```python
from build123d import *

# Parameters (mm, degrees)
BASE_PLATE_R        = 1.6
EXTRUDE_1_DEPTH     = 6
CUT_EXTRUDE_START   = -6
SKETCH_1_R          = 3.25
SKETCH_1_R_2        = 3.5
CUT_EXTRUDE_1_DEPTH = 4.5
SKETCH_1_6_R        = 2.4
CUT_EXTRUDE_2_DEPTH = 2
SKETCH_1_7_R        = 2.5
CUT_EXTRUDE_3_DEPTH = 1.4
FILLET_2_R          = 0.5


with BuildPart() as part:
    # Base plate → 凸台-拉伸1 (new body)
    with BuildSketch(Plane(origin=(0, 0, 0), x_dir=(1, 0, 0), z_dir=(0, 1, 0))):
        with BuildLine():
            Line((-38.1, -38.1), (38.1, -38.1))
            Line((38.1, -38.1), (38.1, 38.1))
            Line((38.1, 38.1), (-0.9, 38.1))
            Line((-0.9, 38.1), (-0.9, 27.4))
            ThreePointArc((-0.9, 27.4), (-2.9, 25.4), (-4.9, 27.4))
            Line((-4.9, 27.4), (-4.9, 38.1))
            Line((-4.9, 38.1), (-38.1, 38.1))
            Line((-38.1, 38.1), (-38.1, -38.1))
        make_face()
        with Locations(Location((-33.9, -33.9, 0), (0, 0, 270))):
            Circle(BASE_PLATE_R, mode=Mode.SUBTRACT)
        with Locations(Location((33.9, -33.9, 0), (0, 0, 270))):
            Circle(BASE_PLATE_R, mode=Mode.SUBTRACT)
        with Locations(Location((-33.9, 33.9, 0), (0, 0, 270))):
            Circle(BASE_PLATE_R, mode=Mode.SUBTRACT)
        with Locations(Location((33.9, 33.9, 0), (0, 0, 270))):
            Circle(BASE_PLATE_R, mode=Mode.SUBTRACT)
    extrude(amount=EXTRUDE_1_DEPTH)

    # 草图1 → 切除-拉伸1 (cut)
    with BuildSketch(Plane.XZ.offset(CUT_EXTRUDE_START)):
        with Locations(Location((-0.35, 10.415, 0), (0, 0, 90))):
            Circle(SKETCH_1_R)
        with Locations(Location((-22.7, 23.9, 0), (0, 0, 90))):
            Circle(SKETCH_1_R)
        with Locations(Location((-22.7, -3.07, 0), (0, 0, 90))):
            Circle(SKETCH_1_R)
        with Locations(Location((-17.96, -15.36, 0), (0, 0, 90))):
            Circle(SKETCH_1_R_2)
        with Locations(Location((-5.01, -15.36, 0), (0, 0, 90))):
            Circle(SKETCH_1_R_2)
    extrude(amount=CUT_EXTRUDE_1_DEPTH, mode=Mode.SUBTRACT)

    # 草图1<6> → 切除-拉伸2 (cut)
    with BuildSketch(Plane.XZ.offset(CUT_EXTRUDE_START)):
        with BuildLine():
            Line((8.9, 2), (8.9, -7.4))
            ThreePointArc((8.9, -7.4), (11.4, -9.9), (13.9, -7.4))
            Line((13.9, -7.4), (13.9, 2))
            ThreePointArc((13.9, 2), (11.4, 4.5), (8.9, 2))
        make_face()
        with BuildLine():
            Line((21.6, -0.16), (21.6, -5.24))
            ThreePointArc((21.6, -5.24), (24.1, -7.74), (26.6, -5.24))
            Line((26.6, -5.24), (26.6, -0.16))
            ThreePointArc((26.6, -0.16), (24.1, 2.34), (21.6, -0.16))
        make_face()
        with Locations(Location((31.9, -15.1, 0), (0, 0, 90))):
            Circle(SKETCH_1_6_R)
        with Locations(Location((16.7, -15.1, 0), (0, 0, 90))):
            Circle(SKETCH_1_6_R)
    extrude(amount=CUT_EXTRUDE_2_DEPTH, mode=Mode.SUBTRACT)

    # 草图1<7> → 切除-拉伸3 (cut)
    with BuildSketch(Plane.XZ.offset(CUT_EXTRUDE_START)):
        with BuildLine():
            Line((17.15, -38.1), (21.65, -38.1))
            Line((21.65, -38.1), (21.65, -37.1))
            Line((21.65, -37.1), (21.65, -36.1))
            ThreePointArc((21.65, -36.1), (20.560909108, -34.172620939), (18.347964405, -34.111100529))
            ThreePointArc((18.347964405, -34.111100529), (17.472620939, -34.939090892), (17.15, -36.1))
            Line((17.15, -36.1), (17.15, -38.1))
        make_face()
        with BuildLine():
            Line((21.65, -36.1), (21.65, -37.1))
            Line((21.65, -37.1), (25.452035595, -35.088899471))
            ThreePointArc((25.452035595, -35.088899471), (23.239090892, -35.027379061), (22.15, -33.1))
            Line((22.15, -33.1), (22.15, -32.1))
            Line((22.15, -32.1), (18.347964405, -34.111100529))
            ThreePointArc((18.347964405, -34.111100529), (20.560909108, -34.172620939), (21.65, -36.1))
        make_face()
        with BuildLine():
            ThreePointArc((22.15, -33.1), (24.4, -35.35), (26.65, -33.1))
            Line((26.65, -33.1), (26.65, -28.1))
            ThreePointArc((26.65, -28.1), (24.4, -25.85), (22.15, -28.1))
            Line((22.15, -28.1), (22.15, -33.1))
        make_face()
        with BuildLine():
            Line((18.347964405, -27.088899471), (22.15, -29.1))
            Line((22.15, -29.1), (22.15, -28.1))
            ThreePointArc((22.15, -28.1), (23.239090892, -26.172620939), (25.452035595, -26.111100529))
            Line((25.452035595, -26.111100529), (22.211102988, -24.396797462))
            Line((22.211102988, -24.396797462), (21.438912065, -26.051492297))
            ThreePointArc((21.438912065, -26.051492297), (20.115915291, -27.233064766), (18.347964405, -27.088899471))
        make_face()
        with BuildLine():
            Line((18.761087935, -21.148507703), (17.361087935, -24.148507703))
            ThreePointArc((17.361087935, -24.148507703), (18.448507703, -27.138912065), (21.438912065, -26.051492297))
            Line((21.438912065, -26.051492297), (22.838912065, -23.051492297))
            ThreePointArc((22.838912065, -23.051492297), (21.751492297, -20.061087935), (18.761087935, -21.148507703))
        make_face()
        with BuildLine():
            Line((38.1, -20.6), (30.8, -20.6))
            ThreePointArc((30.8, -20.6), (29.3, -22.1), (30.8, -23.6))
            Line((30.8, -23.6), (38.1, -23.6))
            Line((38.1, -23.6), (38.1, -20.6))
        make_face()
        with BuildLine():
            Line((17.1, 21.71), (17.1, 14.09))
            ThreePointArc((17.1, 14.09), (19.6, 11.59), (22.1, 14.09))
            Line((22.1, 14.09), (22.1, 21.71))
            ThreePointArc((22.1, 21.71), (19.6, 24.21), (17.1, 21.71))
        make_face()
        with Locations(Location((27.7, 17.9, 0), (0, 0, 90))):
            Circle(SKETCH_1_7_R)
    extrude(amount=CUT_EXTRUDE_3_DEPTH, mode=Mode.SUBTRACT)

    # 圆角2
    fillet_2_edges = [part.edges().sort_by_distance(p)[0] for p in [
        (38.1, 5.3, -23.6),
        (38.1, 5.3, -20.6),
        (21.65, 5.3, -38.1),
        (21.65, 5.3, -37.1),
        (22.211102988, 5.3, -24.396797462),
        (22.15, 5.3, -29.1),
        (22.15, 5.3, -32.1),
        (17.15, 5.3, -38.1),
    ]]
    fillet(fillet_2_edges, radius=FILLET_2_R)


solid = part.part
```
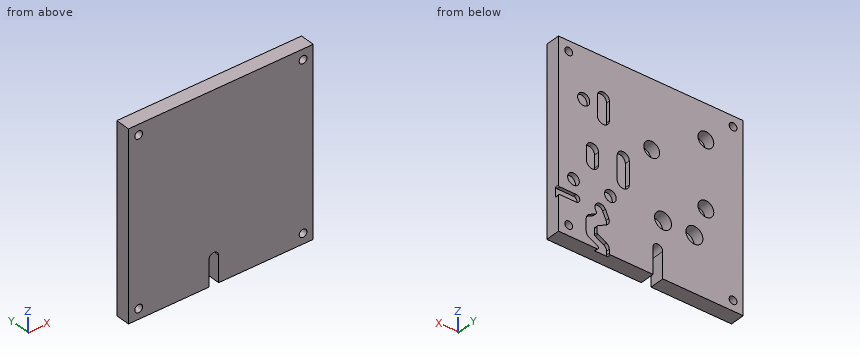
Check sheet for the modelled part. Datum: model origin and axes. Units: mm. Give positions to 0.01 mm unless a question says otherwise; leave off trailing zeros. Order: outer loops, then holes, each group sorted by start corner. A loop starts at its lowest first (then second) coordinate and runs counter-clockwise, first axis right, second up. Notation, with made-up numbers: M 62,35 L 116,35 A19 ccw 116,45 Z; hole C -25.75,1 d1. An arc over 180 degrees is marked long. Answer in a Markdown table with one row per item. Add a question column.
Q1. Sectioned sample at B-B, the plane x = -22.7. Record the boundary of the cut face in (y, z), and give its area (3 significant figures).
Q2. Thickness scan on L1, parallel to Z at x = -22.7, y = 3.7; L2, parallel to X at y = 3.4, z = -33.9; L3, parallel to X at y = 5.1, z = -15.1. Record the ranges inside material, lowest first.
Q3. Sectioned sample at D-D, the plane z = -16.5. Record the boundary of the cut face in (x, y).
Q4. Sectioned sample at C-C, the plane z = -2. Record the boundary of the cut face in (x, y).
Q5. Sectioned sample at A-A, the plane z = 17.9. Record the boundary of the cut face in (x, y).
Q6. Gauge pin test, flat ends, axial feed: pin 1 Ø2.5 at (x, z) = (17.5, -14) entering from +Y; pin 2 Ø2.5 at (x, z) = (23, -3) entering from +Y; pin 3 Ø2.5 at (x, z) = (18.5, 19) entering from +Y; pin 4 Ø3 at (x, z) = (-33.9, -33.9) entering from -Y. Record the tip position at first contact, or that the pin passes through.
Verdict:
| question | item | result |
|---|---|---|
| 1 | outline | M 0,-38.1 L 6,-38.1 L 6,-6.32 L 1.5,-6.32 L 1.5,0.18 L 6,0.18 L 6,20.65 L 1.5,20.65 L 1.5,27.15 L 6,27.15 L 6,38.1 L 0,38.1 Z |
| 1 | area | 399 mm² |
| 2 | L1 | -38.1 to -6.32, 0.18 to 20.65, 27.15 to 38.1 |
| 2 | L2 | -38.1 to -35.5, -32.3 to -4.9, -0.9 to 32.3, 35.5 to 38.1 |
| 2 | L3 | -38.1 to -21.45, -14.47 to -8.5, -1.52 to 14.3, 19.1 to 29.5, 34.3 to 38.1 |
| 3 | outline | M -38.1,0 L 38.1,0 L 38.1,6 L 33.85,6 L 33.85,4 L 29.95,4 L 29.95,6 L 18.65,6 L 18.65,4 L 14.75,4 L 14.75,6 L -1.7,6 L -1.7,1.5 L -8.32,1.5 L -8.32,6 L -14.65,6 L -14.65,1.5 L -21.27,1.5 L -21.27,6 L -38.1,6 Z |
| 4 | outline | M -38.1,0 L 38.1,0 L 38.1,6 L 26.6,6 L 26.6,4 L 21.6,4 L 21.6,6 L 13.9,6 L 13.9,4 L 8.9,4 L 8.9,6 L -19.63,6 L -19.63,1.5 L -25.77,1.5 L -25.77,6 L -38.1,6 Z |
| 5 | outline | M -38.1,0 L 38.1,0 L 38.1,6 L 30.2,6 L 30.2,4.6 L 25.2,4.6 L 25.2,6 L 22.1,6 L 22.1,4.6 L 17.1,4.6 L 17.1,6 L -38.1,6 Z |
| 6 | pin 1 | y = 6 |
| 6 | pin 2 | y = 4 |
| 6 | pin 3 | y = 4.6 |
| 6 | pin 4 | through |
